Check sheet for the drawn part. Datum: minimum x, y, z corner. Units: mm. Coordinates: 2 decimals unless noted, no trailing zeros. Write each loop counter-clockwise with the first axis right and the second up, starting at its lowest first coordinate (ties: lowest second). Pieces come first, ordered by that corner, then holes. Notation, with made-up numbers: M 10,36.5 L 60,36.5 A16 ccw 60,65.5 Z; hole C 61,82 d5. An arc over 180 degrees is marked long. Answer in a Markdown table with one row per item.
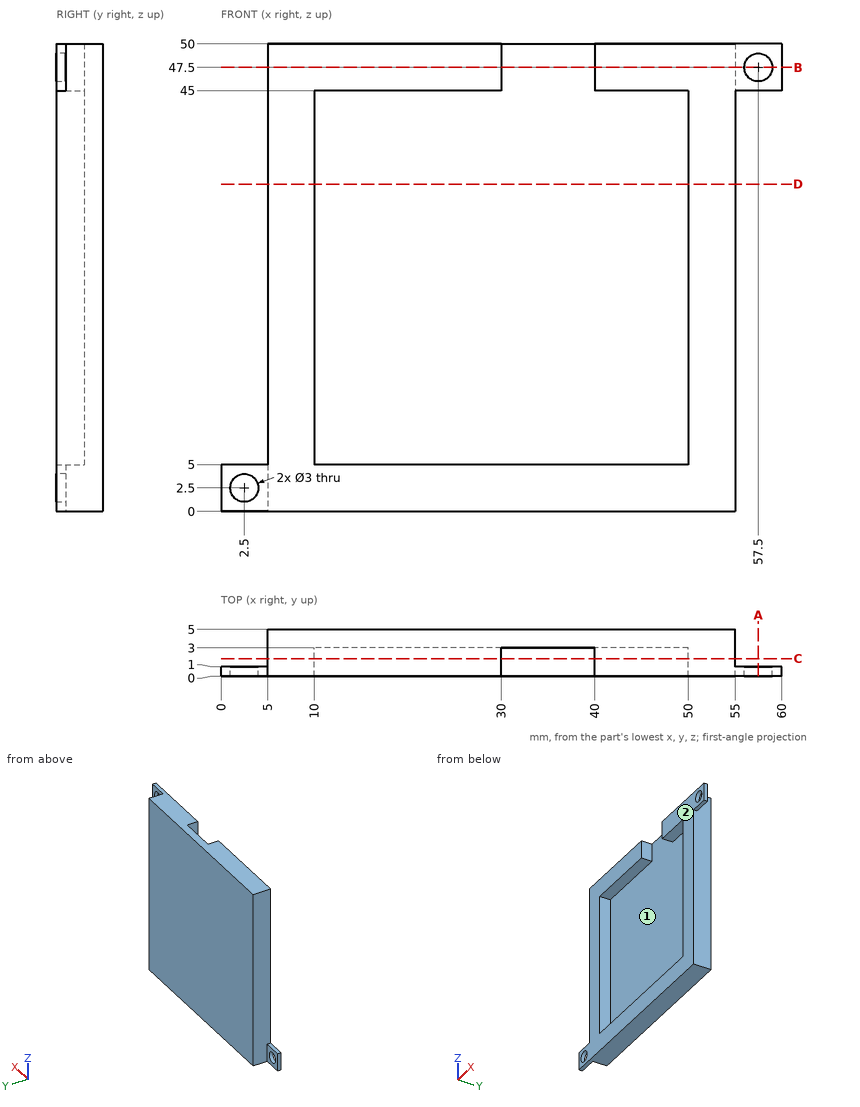
1) Depth check by flat-ended pin: pin 1 (1.5 mm diameter, centred on y = 1, z = 16, fed in from -X); pin 2 (0.5 mm diameter, centred on x = 2.5, y = 0.5, fed in from +Z); pin 3 (0.9 mm diameter, centred on x = 43, y = 1.5, fed in from -Z); pin 4 (0.5 mm diameter, centred on x = 57, y = 0.5, fed in from -Z). Enter the tip coordinate at first touch or a pass-through.
Response values:
| item | result |
|---|---|
| pin 1 | stops at x = 5 |
| pin 2 | stops at z = 5 |
| pin 3 | stops at z = 0 |
| pin 4 | stops at z = 45 |
2) Release check for a two-part mould opening along X. For the marked faces 1 and 2 record: +X half, -X half, draft (parallel to the pull), parting line (faces both ways), or undercut.
Response values:
| item | result |
|---|---|
| face 1 | undercut |
| face 2 | draft |
3) Sectioned sample at C-C (y = 1.85). Record the cut outline in (x, z).
Response values:
| item | result |
|---|---|
| outline | M 5,0 L 55,0 L 55,50 L 40,50 L 40,45 L 50,45 L 50,5 L 10,5 L 10,45 L 30,45 L 30,50 L 5,50 Z |
4) Sectioned sample at D-D (z = 35). Record the cut outline in (x, y), then the cut area to 3 significant figures.
Response values:
| item | result |
|---|---|
| outline | M 5,0 L 10,0 L 10,3 L 50,3 L 50,0 L 55,0 L 55,5 L 5,5 Z |
| area | 130 mm² |
5) Sectioned sample at A-A (x = 57.5). Record the cut outline in (y, z).
Response values:
| item | result |
|---|---|
| outline | M 0,45 L 1,45 L 1,46 L 0,46 Z; M 0,49 L 1,49 L 1,50 L 0,50 Z |
6) Sectioned sample at B-B (z = 47.5). Record the cut outline in (x, y), then the cut area to 3 significant figures.
Response values:
| item | result |
|---|---|
| outline | M 5,0 L 30,0 L 30,3 L 40,3 L 40,0 L 56,0 L 56,1 L 55,1 L 55,5 L 5,5 Z; M 59,0 L 60,0 L 60,1 L 59,1 Z |
| area | 222 mm² |
7) Thickness scan on L1, parallel to X at y = 0.35, z = 47.5; L2, parallel to Z at x = 25.5, y = 2.95; L3, parallel to X at y = 0.75, z = 2.5. Record the ranges inside material, lowest first. Write a range as [from, to].
Response values:
| item | result |
|---|---|
| L1 | x = [5, 30], [40, 56], [59, 60] |
| L2 | z = [0, 5], [45, 50] |
| L3 | x = [0, 1], [4, 55] |
